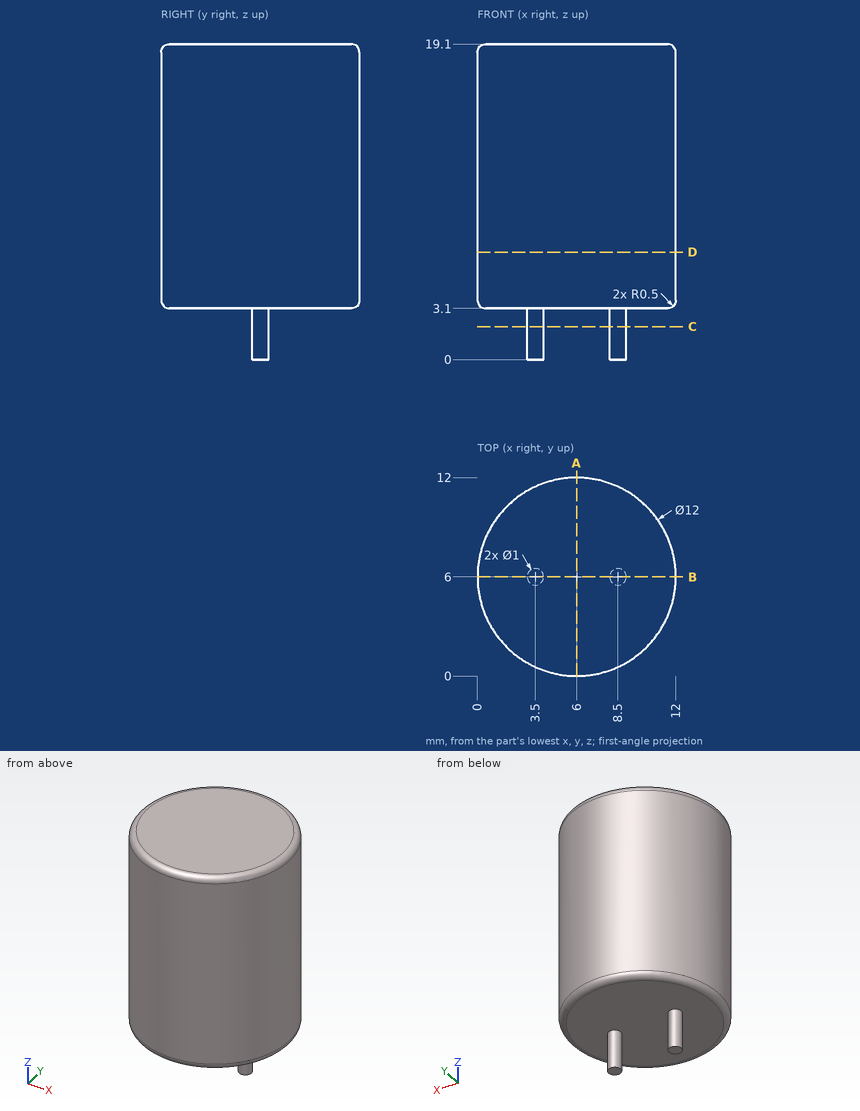
Could you check a few things on this drawing? It's one solid part, dimensions in mm from its lowest x, y, z. Give positions to 0.01 mm unless a question says otherwise; leave off trailing zeros. Loops run counter-clockwise (first coordinate to the right, second up) from the corner with the lowest first, then second, coordinate; pieces in that order, holes last. Notation, with made-up numbers: M 79,-10.5 L 113,-10.5 A14 cw 113,6.5 Z; hole C 4.25,76 d3. An arc over 180 degrees is marked long. Answer as a JSON object with one key per item and string values.
Q1. Suppose I cut it at A-A, the plane x = 6. List the corners of the cut face in (y, z) for me.
Values found:
{"outline": "M 0,3.6 A0.5 ccw 0.5,3.1 L 11.5,3.1 A0.5 ccw 12,3.6 L 12,18.6 A0.5 ccw 11.5,19.1 L 0.5,19.1 A0.5 ccw 0,18.6 Z"}
Q2. Suppose I cut it at C-C, the plane z = 2. List the corners of the cut face in (x, y) for me, plus the area to 3 significant figures.
Values found:
{"outline": "C 3.5,6 d1; C 8.5,6 d1", "area": "1.57 mm²"}
Q3. For P1, Ø4, axis at x = 3.5, z = 17, coming from the -Y side; P2, Ø1, axis at y = 1, z = 8, coming from the +X side; P3, Ø2, axis at x = 8, z = 14, coming from the +Y side, each with a flat end and sliding along its axis, tell me the tip position at first contact or that it passes through.
Values found:
{"P1": "stops at y = 0.02", "P2": "stops at x = 9.97", "P3": "stops at y = 11.92"}
Q4. Suppose I cut it at B-B, the plane y = 6. List the corners of the cut face in (x, z) for me, plus the area to 3 significant figures.
Values found:
{"outline": "M 0,3.6 A0.5 ccw 0.5,3.1 L 3,3.1 L 3,0 L 4,0 L 4,3.1 L 8,3.1 L 8,0 L 9,0 L 9,3.1 L 11.5,3.1 A0.5 ccw 12,3.6 L 12,18.6 A0.5 ccw 11.5,19.1 L 0.5,19.1 A0.5 ccw 0,18.6 Z", "area": "198 mm²"}
Q5. If I drill on probe 1 along Z at (x, y) = (10.5, 3.75); probe 2 along Y at (x, z) = (6.25, 13.5); probe 3 along Z at (x, y) = (2.5, 1.25), over which ranges is the centre line in solid material (lowest first)? Write a range as [from, to].
Values found:
{"probe 1": "z = [3.1, 19.1]", "probe 2": "y = [0.01, 11.99]", "probe 3": "z = [3.3, 18.9]"}
Q6. Suppose I cut it at D-D, the plane z = 6.5. List the corners of the cut face in (x, y) for me.
Values found:
{"outline": "C 6,6 d12"}
